The model under review builds one solid part; all positions refer to its coordinate system, in mm. A direction names the side the tool comes from. Coordinates: 2 decimals unless noted, no trailing zeros. Order: outer loops, then holes, each group sorted by start corner. A loop starts at its lowest first (then second) coordinate and runs counter-clockwise, first axis right, second up. Notation, with made-up numbers: M 46,-27.5 L 51,-27.5 A20 ccw 51,7.5 Z; hole C -13.75,59 d5. An arc over 180 degrees is marked long. Answer in a Markdown table with one row per item.
Solid Edge part; units mm, degrees
sketch "Sketch1" plane through (0, 0, 0) normal (0, 0, 1) x (1, 0, 0)
  line L0 (-59.9226, -59.9226) -> (59.9226, -59.9226)
  line L1 (59.9226, -59.9226) -> (59.9226, 59.9226)
  line L2 (59.9226, 59.9226) -> (-59.9226, 59.9226)
  line L3 (-59.9226, 59.9226) -> (-59.9226, -59.9226)
extrude "Protrusion1" add sketch "Sketch1" along normal mid plane 60
sketch "Sketch2" plane through (0, 0, 30) normal (0, 0, 1) x (1, 0, 0)
  line L0 (69.8659, -5.8454) -> (15.3093, -5.8454)
  line L1 (15.3093, -5.8454) -> (15.3093, -68.7525)
extrude "Cutout1" cut sketch "Sketch2" against normal through all material side at (42.5876, -5.8954, 30)
fillet "Round_1" radius 20 6 edges at (-59.9226, -59.9226, 0) (-59.9226, 59.9226, 0) (15.3093, -5.8454, 0) (15.3093, -59.9226, 0) (59.9226, -5.8454, 0) (59.9226, 59.9226, 0)
sketch "Sketch3" plane through (15.3093, -39.9226, 30) normal (0, -1, 0) x (1, 0, 0)
  circle A0 centre (0, 0) radius 5
sketch3d "SweptCutout1 path"
  arc A0 (-4.6907, -59.9226, 30) -> (15.3093, -39.9226, 30) centre (-4.6907, -39.9226, 30)
  line L1 (15.3093, -25.8454, 30) -> (15.3093, -39.9226, 30)
  arc A2 (15.3093, -25.8454, 30) -> (35.3093, -5.8454, 30) centre (35.3093, -25.8454, 30)
  line L3 (39.9226, -5.8454, 30) -> (35.3093, -5.8454, 30)
  arc A4 (59.9226, 14.1546, 30) -> (39.9226, -5.8454, 30) centre (39.9226, 14.1546, 30)
  line L5 (59.9226, 14.1546, 30) -> (59.9226, 39.9226, 30)
  arc A6 (39.9226, 59.9226, 30) -> (59.9226, 39.9226, 30) centre (39.9226, 39.9226, 30)
  line L7 (39.9226, 59.9226, 30) -> (-39.9226, 59.9226, 30)
  arc A8 (-59.9226, 39.9226, 30) -> (-39.9226, 59.9226, 30) centre (-39.9226, 39.9226, 30)
  line L9 (-59.9226, 39.9226, 30) -> (-59.9226, -39.9226, 30)
  arc A10 (-39.9226, -59.9226, 30) -> (-59.9226, -39.9226, 30) centre (-39.9226, -39.9226, 30)
  line L11 (-39.9226, -59.9226, 30) -> (-4.6907, -59.9226, 30)
sweep "SweptCutout1" cut profiles "Sketch3" path "SweptCutout1 path"
(1) Insertion check: P1, Ø1.4, axis at x = 36.5, z = 6.5, coming from the -Y side; P2, Ø7, axis at y = -33.5, z = 2.5, coming from the +X side. Each pin has a flat end and moves straight along its axis. Give the tip position at first contact, or say it passes through.
Report:
| item | result |
|---|---|
| P1 | y = -5.85 |
| P2 | x = 15.31 |
(2) Machinability: for faces 1 (the flat face through (38, -5.845, -2)), 2 (the cylindrical face through (-56.426, -0.559, 26.426)), 3 (the cylindrical face through (37.648, -2.349, 26.426)), which of the approach directions +Z, -Z, +X, -X, +Y, -Y give a long, thin tool a straight path to every point of the face, cutting with its end or side? Answer none if there is none.
Report:
| item | result |
|---|---|
| face 1 | +Z, -Z, +X, -Y |
| face 2 | +Z, -X, +Y, -Y |
| face 3 | +Z, +X, -Y |
(3) To check wall thickness, follow line 1 (X direction, y = -38.5, z = 4); line 2 (Y direction, x = -4.5, z = 16.5); line 3 (Y direction, x = 36.5, z = 5). State the ranges of each line that lie inside material, in increasing order. Write a range as [from, to].
Report:
| item | result |
|---|---|
| line 1 | [-59.92, 15.31] |
| line 2 | [-59.92, 59.92] |
| line 3 | [-5.85, 59.92] |
(4) Take a section at A-A (z = 18.5). Write out the cut boundary in (x, y), then the cut area to 3 significant figures.
Report:
| item | result |
|---|---|
| outline | M -59.92,-39.92 A20 ccw -39.92,-59.92 L -4.69,-59.92 A20 ccw 15.31,-39.92 L 15.31,-25.85 A20 cw 35.31,-5.85 L 39.92,-5.85 A20 ccw 59.92,14.15 L 59.92,39.92 A20 ccw 39.92,59.92 L -39.92,59.92 A20 ccw -59.92,39.92 Z |
| area | 11,600 mm^2 |
(5) The part is to be moulded in two halves that separate along Z. For faces 4 (the cylindrical face through (11.81, -32.79, 26.43)), 5 (the cylindrical face through (54.22, 53.91, -2.11)), 6 (the flat face through (-1, 1, -30)), say which applies: +Z half, -Z half, draft (parallel to the pull), parting line (faces both ways), or undercut.
Report:
| item | result |
|---|---|
| face 4 | +Z half |
| face 5 | draft |
| face 6 | -Z half |
